Model file for the job. Use its own axes, mm. A direction names the side the tool comes from. Give positions to 0.01 mm unless a question says otherwise; leave off trailing zeros. Loops run counter-clockwise (first coordinate to the right, second up) from the corner with the lowest first, then second, coordinate; pieces in that order, holes last. Notation, with made-up numbers: (54.25, 11.25) - (113.25, 11.25) arc R33 ccw to (113.25, 50.25) - close; hole circle Ø3 at (75.25, 56). An arc over 180 degrees is marked (long way). Use a Markdown table: item, result.
from build123d import *

# Parameters (mm, degrees)
EXTRUDE_1_DEPTH               = 9
SKETCH_2_W                    = 12
SKETCH_2_H                    = 16
CUT_EXTRUDE_1_DEPTH           = 24
HOLE_WIZARD_4_8_1_D           = 6.6
HOLE_WIZARD_4_8_1_CBORE_D     = 11
HOLE_WIZARD_4_8_1_CBORE_DEPTH = 4.7
FILLET_1_R                    = 2


with BuildPart() as part:
    # 草图1 → 凸台-拉伸1 (new, symmetric)
    with BuildSketch(Plane.XY):
        Polygon((0, 0), (-12, 0), (-36, 16.5), (-36, 92.5), (-12, 109), (0, 109), (0, 90), (-30, 90), (-30, 19), (0, 19), align=None)
    extrude(amount=EXTRUDE_1_DEPTH, both=True)

    # 草图2 → 切除-拉伸1 (cut)
    with BuildSketch(Plane.ZY.offset(36)):
        with Locations((0, 101)):
            Rectangle(SKETCH_2_W, SKETCH_2_H)
    cut_extrude_1 = extrude(amount=-CUT_EXTRUDE_1_DEPTH, mode=Mode.SUBTRACT)

    # 打孔尺寸根据内六角花形圆柱头螺钉-4.8级的类型1 (through all)
    with Locations(Plane.ZY.offset(12)):
        with Locations((0, 99.5)):
            hole_wizard_4_8_1 = CounterBoreHole(HOLE_WIZARD_4_8_1_D / 2, HOLE_WIZARD_4_8_1_CBORE_D / 2, HOLE_WIZARD_4_8_1_CBORE_DEPTH)

    # 镜向1: 切除-拉伸1, 打孔尺寸根据内六角花形圆柱头螺钉-4.8级的类型1 across plane
    add(cut_extrude_1.mirror(Plane.ZX.offset(54.5)), mode=Mode.SUBTRACT)
    add(hole_wizard_4_8_1.mirror(Plane.ZX.offset(54.5)), mode=Mode.SUBTRACT)

    # 圆角1
    # the kernel refuses this fillet: 2 mm, written as the material it takes off along each edge
    with BuildSketch(Plane(origin=(-34, 91.44793902, -7), x_dir=(-1, 0, 0), z_dir=(0, 0, -1))) as fillet_1_piece_1_section:
        Polygon((0, 0), (FILLET_1_R, 0), (FILLET_1_R, FILLET_1_R * 0.526030489934), (FILLET_1_R * 0.566528822887, FILLET_1_R * 0.824041924199), align=None)
    fillet_1_piece_1 = extrude(amount=FILLET_1_R, mode=Mode.PRIVATE)
    fillet_1_piece_1 = fillet_1_piece_1 - Plane(origin=(-34, 91.44793902, -7), x_dir=(0.8850222660721778, -0.46554869622464556, 0), z_dir=(0, 0, -1)) * Sphere(FILLET_1_R, mode=Mode.PRIVATE)
    add(fillet_1_piece_1, mode=Mode.SUBTRACT)
    with BuildSketch(Plane(origin=(-34, 91.44793902, 7), x_dir=(-1, 0, 0), z_dir=(0, 0, 1))) as fillet_1_piece_2_section:
        Polygon((0, 0), (FILLET_1_R, 0), (FILLET_1_R, -FILLET_1_R * 0.526030489934), (FILLET_1_R * 0.566528822887, -FILLET_1_R * 0.824041924199), align=None)
    fillet_1_piece_2 = extrude(amount=FILLET_1_R, mode=Mode.PRIVATE)
    fillet_1_piece_2 = fillet_1_piece_2 - Plane(origin=(-34, 91.44793902, 7), x_dir=(0.8850222660721778, -0.46554869622464556, 0), z_dir=(0, 0, 1)) * Sphere(FILLET_1_R, mode=Mode.PRIVATE)
    add(fillet_1_piece_2, mode=Mode.SUBTRACT)
    with BuildSketch(Plane(origin=(-34, 17.55206098, 7), x_dir=(-1, 0, 0), z_dir=(0, 0, 1))) as fillet_1_piece_3_section:
        Polygon((0, 0), (FILLET_1_R, 0), (FILLET_1_R, FILLET_1_R * 0.526030489934), (FILLET_1_R * 0.566528822887, FILLET_1_R * 0.824041924199), align=None)
    fillet_1_piece_3 = extrude(amount=FILLET_1_R, mode=Mode.PRIVATE)
    fillet_1_piece_3 = fillet_1_piece_3 - Plane(origin=(-34, 17.55206098, 7), x_dir=(0.8850222660721778, 0.46554869622464556, 0), z_dir=(0, 0, 1)) * Sphere(FILLET_1_R, mode=Mode.PRIVATE)
    add(fillet_1_piece_3, mode=Mode.SUBTRACT)
    with BuildSketch(Plane(origin=(-34, 17.55206098, -7), x_dir=(-0.5665288228870655, -0.8240419241993675, 0), z_dir=(0, 0, -1))) as fillet_1_piece_4_section:
        Polygon((0, 0), (FILLET_1_R, 0), (FILLET_1_R, FILLET_1_R * 0.526030489934), (FILLET_1_R * 0.566528822887, FILLET_1_R * 0.824041924199), align=None)
    fillet_1_piece_4 = extrude(amount=FILLET_1_R, mode=Mode.PRIVATE)
    fillet_1_piece_4 = fillet_1_piece_4 - Plane(origin=(-34, 17.55206098, -7), x_dir=(0.8850222660721778, 0.46554869622464556, 0), z_dir=(0, 0, -1)) * Sphere(FILLET_1_R, mode=Mode.PRIVATE)
    add(fillet_1_piece_4, mode=Mode.SUBTRACT)
    with BuildSketch(Plane(origin=(-35.133057646, 93.096022869, -9), x_dir=(0.5665288228870655, -0.8240419241993674, 0), z_dir=(0.8240419241993675, 0.5665288228870655, 0)), Plane(origin=(-7.879790379, -2.832644114, 9), x_dir=(0, 0, -1), z_dir=(-0.8240419241993675, 0.5665288228870655, 0)), Plane(origin=(-7.879790379, -2.832644114, -9), x_dir=(0.5665288228870655, 0.8240419241993675, 0), z_dir=(-0.8240419241993675, 0.5665288228870655, 0))) as fillet_1_piece_5:
        with BuildLine():
            CenterArc((FILLET_1_R, -FILLET_1_R), FILLET_1_R, 90, 90)
            Line((0, -FILLET_1_R), (0, 0))
            Line((0, 0), (FILLET_1_R, 0))
        make_face()
    extrude(amount=33.072670779, mode=Mode.SUBTRACT)
    with BuildSketch(Plane(origin=(-35.133057646, 93.096022869, 9), x_dir=(0.5665288228870655, -0.8240419241993674, 0), z_dir=(0.8240419241993675, 0.5665288228870655, 0))) as fillet_1_piece_6:
        with BuildLine():
            CenterArc((FILLET_1_R, FILLET_1_R), FILLET_1_R, 180, 90)
            Line((0, FILLET_1_R), (0, 0))
            Line((0, 0), (FILLET_1_R, 0))
        make_face()
    extrude(amount=33.072670779, mode=Mode.SUBTRACT)
    with BuildSketch(Plane(origin=(-36, 92.5, 7), x_dir=(0, -1, 0), z_dir=(0, 0, -1)), Plane(origin=(-36, 16.5, 7), x_dir=(0.8240419241993692, -0.566528822887063, 0), z_dir=(0, 0, -1))) as fillet_1_piece_7:
        with BuildLine():
            CenterArc((FILLET_1_R * 0.526030489934, -FILLET_1_R), FILLET_1_R, 90, 55.491477012)
            Line((-FILLET_1_R * 0.298011434265, -FILLET_1_R * 0.433471177113), (0, 0))
            Line((0, 0), (FILLET_1_R * 0.526030489934, 0))
        make_face()
    extrude(amount=14, mode=Mode.SUBTRACT)
    with BuildSketch(Plane(origin=(-36, 17.55206098, -9), x_dir=(1, 0, 0), z_dir=(0, 1, 0))) as fillet_1_piece_8:
        with BuildLine():
            CenterArc((FILLET_1_R, -FILLET_1_R), FILLET_1_R, 90, 90)
            Line((0, -FILLET_1_R), (0, 0))
            Line((0, 0), (FILLET_1_R, 0))
        make_face()
    extrude(amount=73.89587804, mode=Mode.SUBTRACT)
    with BuildSketch(Plane(origin=(-36, 17.55206098, 9), x_dir=(1, 0, 0), z_dir=(0, 1, 0))) as fillet_1_piece_9:
        with BuildLine():
            CenterArc((FILLET_1_R, FILLET_1_R), FILLET_1_R, 180, 90)
            Line((0, FILLET_1_R), (0, 0))
            Line((0, 0), (FILLET_1_R, 0))
        make_face()
    extrude(amount=73.89587804, mode=Mode.SUBTRACT)


solid = part.part
(1) Mould opens along Z. For faces 1 (the flat face through (-36, 54, 0)), 2 (the cylindrical face through (-9.683, 104.953, -0.716)), 3 (the cylindrical face through (-22.21, 101.25, -8.43)), 4 (the flat face through (-7.3, 96, 0)) say: pulls with the +Z half, pulls with the -Z half, needs draft (parallel to the pull), parting line crosses it, or undercut.
Computed:
| item | result |
|---|---|
| face 1 | needs draft |
| face 2 | undercut |
| face 3 | pulls with the -Z half |
| face 4 | undercut |
(2) Slice it at B-B, the plane y = 53. Write the cut outline in (x, z).
Computed:
| item | result |
|---|---|
| outline | (-36, -7) arc R2 ccw to (-34, -9) - (-30, -9) - (-30, 9) - (-34, 9) arc R2 ccw to (-36, 7) - close |
(3) Pin check, flat tips, straight feed: P1, Ø3.5, axis at y = 99, z = 0.5, coming from the -X side; P2, Ø5.5, axis at x = -16, z = -2, coming from the -Y side; P3, Ø9.5, axis at y = 103.5, z = -0.5, coming from the -X side; P4, Ø6, axis at y = 80, z = 3, coming from the +X side. Stop position of each tip, or through.
Computed:
| item | result |
|---|---|
| P1 | through |
| P2 | y = 16 |
| P3 | x = -12 |
| P4 | x = -30 |
(4) Slice it at A-A, the plane z = 0. Count the separate pieces of the cut face and the enclosed holes in it, plus the area to 3 significant figures.
Computed:
| item | result |
|---|---|
| separate pieces | 3 |
| enclosed holes | 0 |
| area | 826 mm² |
(5) Drill centre lines: probe 1 along Y at (x, z) = (-2, 0.25); probe 2 along Y at (x, z) = (-8.4, 0); probe 3 along Z at (x, y) = (-10.95, 9.5). Where is each one in solid material? Low to high. Write a range as [from, to].
Computed:
| item | result |
|---|---|
| probe 1 | [0, 6.21], [12.79, 19], [90, 96.21], [102.79, 109] |
| probe 2 | [0, 4], [15, 19], [90, 94], [105, 109] |
| probe 3 | [-9, -5.5], [5.5, 9] |
(6) 3-axis set-ups, long thin cutter, end or side, ignore diameter. For faces 5 (the flat face through (-23.728, 100.937, -6.493)), 6 (the flat face through (-30, 55, 0)), 7 (the flat face through (-12, 105, -3)), 8 (the flat face through (-24, 16, 0)): which of +Z, -Z, +X, -X, +Y, -Y reach the whole face in a straight line?
Computed:
| item | result |
|---|---|
| face 5 | +Z, -Z, -X, +Y |
| face 6 | +Z, -Z, +X |
| face 7 | -X, +Y |
| face 8 | -X, -Y |
